```python
from build123d import *
from build123d.topology import SkipClean

# Parameters (mm, degrees)
SKETCH5_W           = 100
SKETCH5_H           = 130
BOSS_EXTRUDE1_DEPTH = 150
CUT_EXTRUDE1_START  = -50
CUT_EXTRUDE1_DEPTH  = 40
BOSS_EXTRUDE3_START = 30
SKETCH17_W          = 80
SKETCH17_H          = 40
BOSS_EXTRUDE3_DEPTH = 5
SKETCH10_R          = 8.75
CUT_EXTRUDE3_DEPTH  = 100
SKETCH18_W          = 48.5
SKETCH18_H          = 10
BOSS_EXTRUDE4_DEPTH = 10
BOSS_EXTRUDE5_START = 100
SKETCH18_2_W        = 48.5
SKETCH18_2_H        = 10
BOSS_EXTRUDE5_DEPTH = 10
CUT_EXTRUDE5_DEPTH  = 70
FILLET1_DEPTH       = 10
CUT_EXTRUDE6_DEPTH  = 120
FILLET2_R           = 10
CHAMFER2_SIZE       = 25
BOSS_EXTRUDE6_START = 30
BOSS_EXTRUDE6_DEPTH = 30
FILLET3_R           = 5
CUT_EXTRUDE7_DEPTH  = 5


with BuildPart() as part:
    # Sketch5 → Boss-Extrude1 (new body)
    with BuildSketch(Plane(origin=(0, 0, 0), x_dir=(1, 0, 0), z_dir=(0, 1, 0))):
        with Locations((50, 65)):
            Rectangle(SKETCH5_W, SKETCH5_H)
    extrude(amount=BOSS_EXTRUDE1_DEPTH)

    # Sketch7 → Cut-Extrude1 (cut, symmetric)
    with BuildSketch(Plane(origin=(100, 0, 0), x_dir=(0, 0, -1), z_dir=(1, 0, 0)).offset(CUT_EXTRUDE1_START)):
        Polygon((130, 0), (130, 133.702332435), (0, 42.675352467), (0, 0), align=None)
        Polygon((0, 50), (130, 141.026979967), (130, 150), (0, 150), align=None)
    extrude(amount=CUT_EXTRUDE1_DEPTH, both=True, mode=Mode.SUBTRACT)

    # Sketch17 → Boss-Extrude3 (add)
    with BuildSketch(Plane(origin=(0, 275.412054826, -321.921776796), x_dir=(1, 0, 0), z_dir=(0, -0.819152044288993, -0.5735764363510444)).offset(BOSS_EXTRUDE3_START)):
        with Locations((50, 354.293228142)):
            Rectangle(SKETCH17_W, SKETCH17_H)
    extrude(amount=-BOSS_EXTRUDE3_DEPTH)

    # Sketch10 → Cut-Extrude3 (cut)
    with BuildSketch(Plane(origin=(0, 33.550503583, 23.49231552), x_dir=(1, 0, 0), z_dir=(0, 0.819152044288993, 0.5735764363510444))):
        with Locations(Location((50, 68.178273127, 0), (0, 0, 90))):
            Circle(SKETCH10_R)
    extrude(amount=-CUT_EXTRUDE3_DEPTH, mode=Mode.SUBTRACT)

    # Sketch18 → Boss-Extrude4 (add)
    with BuildSketch(Plane(origin=(0, 0, 0), x_dir=(0, 0, -1), z_dir=(1, 0, 0))):
        with Locations((24.25, 155)):
            Rectangle(SKETCH18_W, SKETCH18_H)
    extrude(amount=BOSS_EXTRUDE4_DEPTH)

    # Sketch18<2> → Boss-Extrude5 (add)
    with BuildSketch(Plane(origin=(0, 0, 0), x_dir=(0, 0, -1), z_dir=(1, 0, 0)).offset(BOSS_EXTRUDE5_START)):
        with Locations((24.25, 155)):
            Rectangle(SKETCH18_2_W, SKETCH18_2_H)
    extrude(amount=-BOSS_EXTRUDE5_DEPTH)

    # Sketch21 → Cut-Extrude5 (cut)
    with BuildSketch(Plane(origin=(0, 0, 0), x_dir=(0, 0, -1), z_dir=(1, 0, 0))):
        Polygon((62.42420648, 63.190535225), (51.526254189, 78.754424066), (18.760172418, 55.811366612), (29.658124708, 40.247477771), align=None)
        Polygon((69.307123716, 53.360710693), (36.541041945, 30.417653239), (32.52600689, 36.151717549), (65.292088662, 59.094775003), align=None)
    extrude(amount=CUT_EXTRUDE5_DEPTH, mode=Mode.SUBTRACT)

    # Fillet1: read off the stored shape, not the designer's step
    # Fillet1 outline → Fillet1 (add)
    with BuildSketch(Plane.YZ):
        with BuildLine():
            Line((30.417653239, -36.541041945), (33.285535421, -40.636802166))
            ThreePointArc((33.285535421, -40.636802166), (32.457256878, -36.900679096), (34.513413461, -33.673159763))
            Line((34.513413461, -33.673159763), (30.417653239, -36.541041945))
        make_face()
        with BuildLine():
            ThreePointArc((43.115359953, -33.75388493), (42.287081409, -30.01776186), (44.343237992, -26.790242527))
            Line((44.343237992, -26.790242527), (40.247477771, -29.658124708))
            Line((40.247477771, -29.658124708), (43.115359953, -33.75388493))
        make_face()
    extrude(amount=FILLET1_DEPTH)

    # Sketch22 → Cut-Extrude6 (cut)
    with BuildSketch(Plane.ZY):
        Polygon((-115, 0), (-95, 20), (-65, 0), align=None)
    extrude(amount=-CUT_EXTRUDE6_DEPTH, mode=Mode.SUBTRACT)

    # Fillet2
    fillet2_edges = [part.edges().sort_by_distance(p)[0] for p in [
        (50, 50, 0),
    ]]
    fillet(fillet2_edges, radius=FILLET2_R)

    # Chamfer2
    chamfer2_edges = [part.edges().sort_by_distance(p)[0] for p in [
        (5, 160, 0),
        (95, 160, 0),
    ]]
    chamfer(chamfer2_edges, length=CHAMFER2_SIZE)

    # Sketch23 → Boss-Extrude6 (add)
    with SkipClean():  # the faces are left unmerged after this step: merging them gives an invalid solid
        with BuildSketch(Plane(origin=(0, 33.550503583, 23.49231552), x_dir=(1, 0, 0), z_dir=(0, 0.819152044288993, 0.5735764363510444)).offset(BOSS_EXTRUDE6_START)):
            with BuildLine():
                Line((90, 90.716932877), (57.180703308, 63.178273127))
                ThreePointArc((57.180703308, 63.178273127), (56.983337112, 62.906129088), (56.77566264, 62.64176739))
                ThreePointArc((56.77566264, 62.64176739), (57.241088602, 60.832062958), (59.109066137, 60.880139798))
                Line((59.109066137, 60.880139798), (90, 86.800711009))
                Line((90, 86.800711009), (90, 90.716932877))
            make_face()
            with BuildLine():
                ThreePointArc((40.890933863, 60.880139798), (42.758911398, 60.832062958), (43.22433736, 62.64176739))
                ThreePointArc((43.22433736, 62.64176739), (43.016662888, 62.906129088), (42.819296692, 63.178273127))
                Line((42.819296692, 63.178273127), (10, 90.716932877))
                Line((10, 90.716932877), (10, 86.800711009))
                Line((10, 86.800711009), (40.890933863, 60.880139798))
            make_face()
        extrude(amount=-BOSS_EXTRUDE6_DEPTH)

    # Fillet3
    fillet3_edges = [part.edges().sort_by_distance(p)[0] for p in [
        (90, 95.624626741, -39.007017804),
        (10, 95.624626741, -39.007017804),
    ]]
    fillet(fillet3_edges, radius=FILLET3_R)

    # Sketch24 → Cut-Extrude7 (cut)
    with SkipClean():  # the faces are left unmerged after this step: merging them gives an invalid solid
        with BuildSketch(Plane(origin=(10, 0, 0), x_dir=(0, 0, -1), z_dir=(1, 0, 0))):
            with BuildLine():
                ThreePointArc((29.577399541, 31.645531279), (36.032438208, 27.533218113), (43.504684348, 29.1897752))
                Line((43.504684348, 29.1897752), (76.270766119, 52.132832654))
                Line((76.270766119, 52.132832654), (69.387848883, 61.962657185))
                Line((69.387848883, 61.962657185), (66.519966701, 66.058417407))
                Line((66.519966701, 66.058417407), (58.489896592, 77.526546027))
                Line((58.489896592, 77.526546027), (125, 124.0974218))
                Line((125, 124.0974218), (125, 5))
                Line((125, 5), (117.071067812, 5))
                Line((117.071067812, 5), (95.637089412, 26.4339784))
                Line((95.637089412, 26.4339784), (63.486121811, 5))
                Line((63.486121811, 5), (5, 5))
                Line((5, 5), (5, 40.072517215))
                Line((5, 40.072517215), (17.532294378, 48.847724209))
                Line((17.532294378, 48.847724209), (22.694482305, 41.475355811))
                Line((22.694482305, 41.475355811), (25.562364487, 37.379595589))
                Line((25.562364487, 37.379595589), (28.430246669, 33.283835368))
                Line((28.430246669, 33.283835368), (29.577399541, 31.645531279))
            make_face()
        cut_extrude7 = extrude(amount=-CUT_EXTRUDE7_DEPTH, mode=Mode.SUBTRACT)

    # Mirror1: Cut-Extrude7 across plane
    with SkipClean():  # the faces are left unmerged after this step: merging them gives an invalid solid
        add(cut_extrude7.mirror(Plane.ZY.offset(-50)), mode=Mode.SUBTRACT)


solid = part.part
```
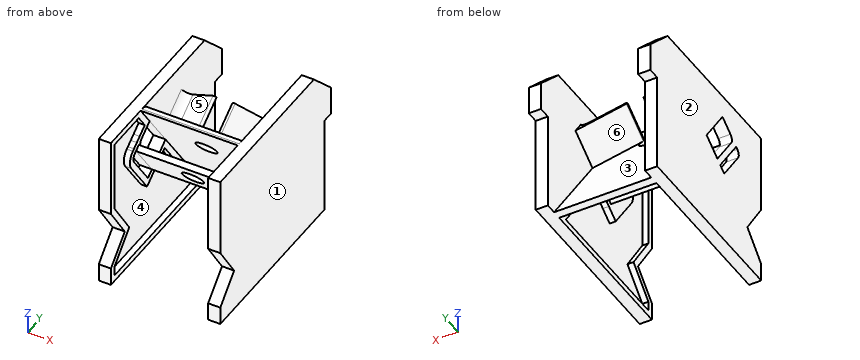
Verification items for the finished model (mm, model axes). Face numbers are marked on the shaded views. A direction names the side the tool comes from. Round coordinates to 2 decimals unless told otherwise and drop trailing zeros. Write each loop counter-clockwise with the first axis right and the second up, starting at its lowest first coordinate (ties: lowest second). Pieces come first, ordered by that corner, then holes. Notation, with made-up numbers: (48.5, 0) - (78.5, 0) arc R28 ccw to (78.5, 26) - close; hole circle Ø3 at (12.5, 17). An arc over 180 degrees is marked (long way). Answer as a JSON object with one key per item and string values. Group by question number.
Q1. Thickness scan on line 1 (X direction, y = 12.5, z = -112); line 2 (X direction, y = 152, z = -19.5); line 3 (Y direction, x = 88, z = -29). Record the ranges inside material, lowest first.
Q2. Go/stop test with flat-tipped pins: pin 1 Ø5 at (x, y) = (6.5, 156.5) entering from -Z; pin 2 Ø1 at (x, z) = (42, -53.5) entering from +Y; pin 3 Ø8 at (x, z) = (96, -88) entering from +Y. Record where each tip stops, or that it passes through.
Q3. Section check C-C, the plane y = 117. Enter the section's corners in (x, z).
Q4. Section check B-B, the plane x = 88. Enter the section's corners in (y, z), plus the area to 3 significant figures.
Q5. Tool access check on the marked faces 4, 5 and 6. Record the directions out of +Z, -Z, +X, -X, +Y, -Y that give a thin tool (end or side, any length) a straight path to the whole face; none if there is none.
Q6. Section check D-D, the plane z = -98. Enter the section's corners in (x, y).
Q7. Mould release check, pull along X, two halves, no side actions. Record for the marked faces 1, 2 and 3: released by +X, released by -X, zero draft, split by the parting line, or undercut.
Q8. Section check A-A, the plane x = 53.5. Enter the section's corners in (y, z), plus the area to 3 significant figures.
Found:
{
 "1": {"line 1": "x = 0 to 5, 95 to 100", "line 2": "x = 0 to 10, 90 to 100", "line 3": "y = 62.98 to 70.31, 98.2 to 106.93"},
 "2": {"pin 1": "stops at z = -48.5", "pin 2": "stops at y = 87.81", "pin 3": "stops at y = 150"},
 "3": {"outline": "(0, -130) - (10, -130) - (10, -125) - (5, -125) - (5, -114.86) - (10, -114.86) - (10, -106.15) - (90, -106.15) - (90, -114.86) - (95, -114.86) - (95, -125) - (90, -125) - (90, -130) - (100, -130) - (100, 0) - (90, 0) - (90, -95.69) - (10, -95.69) - (10, 0) - (0, 0) - close"},
 "4": {"outline": "(36.15, -32.53) - (59.09, -65.29) - (63.19, -62.42) - (40.25, -29.66) - close; (42.68, 0) - (133.7, -130) - (141.03, -130) - (84.62, -49.44) - (109.2, -32.24) - (104.06, -24.9) - (79.48, -42.1) - (52.99, -4.26) arc R10 ccw to (44.79, 0) - close", "area": "1,420 mm^2"},
 "5": {"face 4": "none", "face 5": "+Z", "face 6": "+Y"},
 "6": {"outline": "(0, 17) - (10, 17) - (10, 24.07) - (5, 24.07) - (5, 105.19) - (10, 105.19) - (10, 111.3) - (90, 111.3) - (90, 105.19) - (95, 105.19) - (95, 24.07) - (90, 24.07) - (90, 17) - (100, 17) - (100, 150) - (90, 150) - (90, 118.62) - (10, 118.62) - (10, 150) - (0, 150) - close"},
 "7": {"face 1": "released by +X", "face 2": "released by -X", "face 3": "undercut"},
 "8": {"outline": "(36.15, -32.53) - (43.48, -42.99) - (47.58, -40.13) - (40.25, -29.66) - close; (42.68, 0) - (63.14, -29.23) - (68.06, -25.79) - (52.99, -4.26) arc R10 ccw to (44.79, 0) - close; (52.68, -56.13) - (59.09, -65.29) - (63.19, -62.42) - (56.78, -53.26) - close; (72.34, -42.37) - (133.7, -130) - (141.03, -130) - (77.26, -38.93) - close", "area": "972 mm^2"}
}
